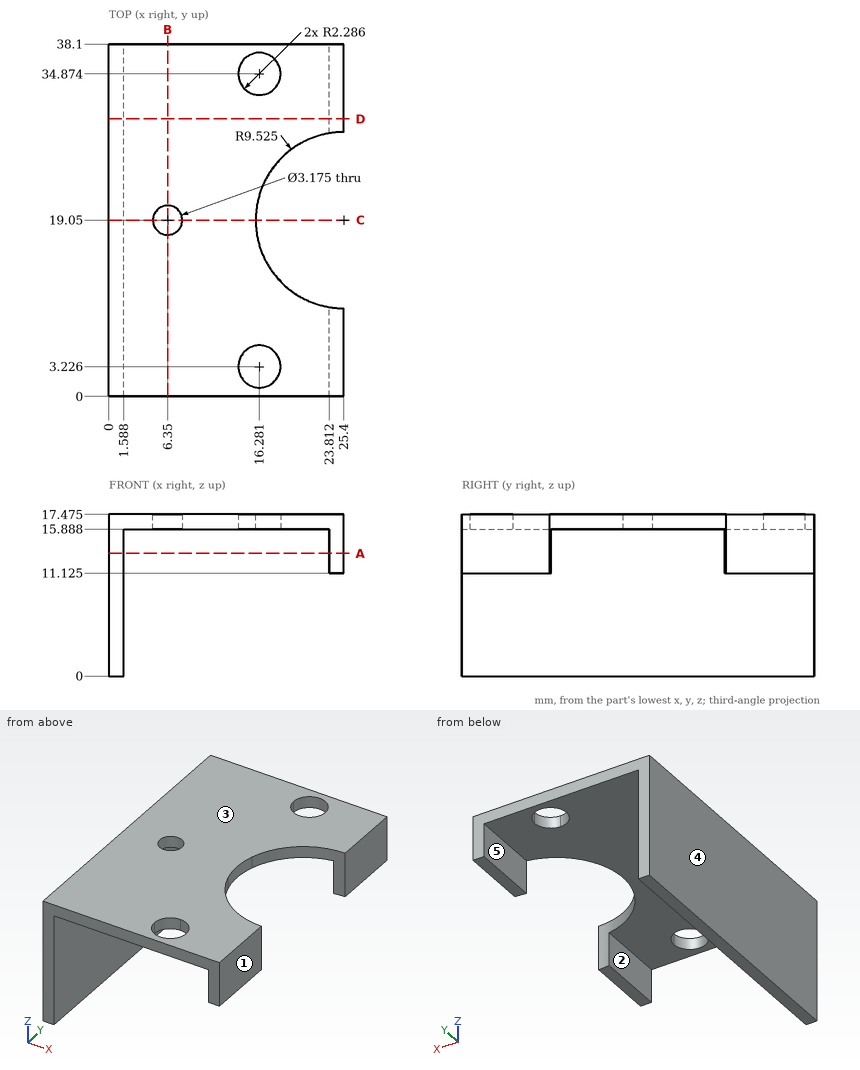
Answer from the drawing. Dimensions are ordinates in mm from the lowest x, y and z of the part. A direction names the side the tool comes from. Round coordinates to 2 decimals unless told otherwise and drop trailing zeros. Loops run counter-clockwise (first coordinate to the right, second up) from the corner with the lowest first, then second, coordinate; pieces in that order, holes last. Notation, with made-up numbers: (67, -21.75) - (122, -21.75) arc R16 ccw to (122, -13.75) - close; hole circle Ø9 at (-18.5, -3). An arc over 180 degrees is marked (long way). Return JSON: item names as keys, results as strings. Group by question number.
1. The part is cut by section D-D on y = 30. Determine the outline of the cut face in (x, z) (1 decimal).
2. Consider probe 1 along Y at (x, z) = (6.35, 16.7); probe 2 along Z at (x, y) = (12.5, 4.5) (1 decimal); probe 3 along X at (y, z) = (20, 11). Determine where each line is inside the solid, lowest interval first.
3. Each of these flat-tipped pins is pushed along its axis until it touches: P1, Ø6.5, axis at x = 14, y = 14.5, coming from the -Z side; P2, Ø1.4, axis at y = 5, z = 14, coming from the -X side; P3, Ø0.8, axis at x = 24.5, y = 7, coming from the -Z side (1 decimal). Where does it stop, or does it pass through?
4. The part is cut by section A-A on z = 13.25. State how many separate pieces and enclosed holes the cut face has.
5. Which of the six approach directions +Z, -Z, +X, -X, +Y, -Y give full straight-line access (tool end or side, diameter ignored) to the marked faces 4 and 5?
6. The part is cut by section B-B on x = 6.35. Determine the outline of the cut face in (y, z) (1 decimal).
7. The part is cut by section C-C on y = 19.05. Determine the outline of the cut face in (x, z) (1 decimal).
8. The mould has two halves that part along X. Classify the marked faces 1, 2 and 3: pulls with the +X half, pulls with the -X half, needs draft (parallel to the pull), parting line crosses it, or undercut.
Resolved:
{
 "1": {"outline": "(0, 0) - (1.6, 0) - (1.6, 15.9) - (23.8, 15.9) - (23.8, 11.1) - (25.4, 11.1) - (25.4, 17.5) - (0, 17.5) - close"},
 "2": {"probe 1": "y = 0 to 17.46, 20.64 to 38.1", "probe 2": "z = 15.9 to 17.5", "probe 3": "x = 0 to 1.59"},
 "3": {"P1": "stops at z = 15.89", "P2": "stops at x = 0", "P3": "stops at z = 11.1"},
 "4": {"separate pieces": "3", "enclosed holes": "0"},
 "5": {"face 4": "+Z, -Z, -X, +Y, -Y", "face 5": "-Z, +Y, -Y"},
 "6": {"outline": "(0, 15.9) - (17.5, 15.9) - (17.5, 17.5) - (0, 17.5) - close; (20.6, 15.9) - (38.1, 15.9) - (38.1, 17.5) - (20.6, 17.5) - close"},
 "7": {"outline": "(0, 0) - (1.6, 0) - (1.6, 15.9) - (4.8, 15.9) - (4.8, 17.5) - (0, 17.5) - close; (7.9, 15.9) - (15.9, 15.9) - (15.9, 17.5) - (7.9, 17.5) - close"},
 "8": {"face 1": "pulls with the +X half", "face 2": "undercut", "face 3": "needs draft"}
}
